Geometry: final body of the model. Coordinates: model frame, mm. Give positions to 0.01 mm unless a question says otherwise; leave off trailing zeros. Loops run counter-clockwise (first coordinate to the right, second up) from the corner with the lowest first, then second, coordinate; pieces in that order, holes last. Notation, with made-up numbers: M 45.25,50.5 L 50.25,50.5 A15 ccw 50.25,62.5 Z; hole C -14.75,-21.75 d8. An arc over 180 degrees is marked long. Put each result on its own line as item: value.
```python
from build123d import *

# Parameters (mm, degrees)
F0_W     = 6.477
F0_H     = 50.8
F1_DEPTH = 25.4


with BuildPart() as f1:
    # F0 (on Right) → F1 (new body)
    with BuildSketch(Plane.YZ):
        Polygon((43.560641, 26.136384), (0, 0), (508, 0), (508, 50.8), (508, 254), (508, 304.8), (464.439359, 278.663616), align=None)
        Polygon((-3.332389, 5.553982), (0, 0), (43.560641, 26.136384), (40.228252, 31.690366), align=None)
        with Locations((511.2385, 25.4)):
            Rectangle(F0_W, F0_H)
        Polygon((461.10697, 284.217597), (464.439359, 278.663616), (508, 304.8), (504.667611, 310.353982), align=None)
        with Locations((511.2385, 279.4)):
            Rectangle(F0_W, F0_H)
    extrude(amount=F1_DEPTH)


solid = f1.part
```
Item 1: Mould query, pull axis Z, two halves, no side actions, for faces 1 (the flat face through (12.522, 483.192, 297.469)), 2 (the flat face through (13, 508, 151)), 3 (the flat face through (0, 367, 88)). Classes: pulls with the +Z half, pulls with the -Z half, needs draft (parallel to the pull), parting line crosses it, or undercut.
Output values:
face 1: pulls with the +Z half
face 2: undercut
face 3: needs draft
Item 2: Pin query (flat end, axial travel): pin 1 Ø12 at (x, z) = (18, 145) entering from -Y; pin 2 Ø12.5 at (x, z) = (12, 199.5) entering from +Y; pin 3 Ø1.9 at (x, y) = (15.5, 512) entering from +Z. Return the tip coordinate at first contact, or that it passes through.
Output values:
pin 1: y = 231.67
pin 2: y = 508
pin 3: z = 304.8
Item 3: Section A-A on x = 14.75. Output: boundary loops of the cut face in (y, z).
Output values:
outline: M -3.33,5.55 L 0,0 L 514.48,0 L 514.48,50.8 L 508,50.8 L 508,254 L 514.48,254 L 514.48,304.8 L 508,304.8 L 504.67,310.35 L 461.11,284.22 L 464.44,278.66 L 43.56,26.14 L 40.23,31.69 Z
Item 4: Line query: probe 1 along Y at (x, z) = (6.5, 229.5); probe 2 along Y at (x, z) = (24.75, 258); probe 3 along Z at (x, y) = (16.25, 207.5). Output: solid intervals per line, ascending. Write a range as [from, to].
Output values:
probe 1: [382.5, 508]
probe 2: [430, 514.48]
probe 3: [0, 124.5]
Item 5: Section B-B on y = 244.5. Output: boundary loops of the cut face in (x, z).
Output values:
outline: M 0,0 L 25.4,0 L 25.4,146.7 L 0,146.7 Z
Item 6: Section C-C on z = 226.5. Output: boundary loops of the cut face in (x, y).
Output values:
outline: M 0,377.5 L 25.4,377.5 L 25.4,508 L 0,508 Z
